from build123d import *

# Parameters (mm, degrees)
PAD_DEPTH          = 1.5
SKETCH001_R        = 2.9
PAD001_DEPTH       = 2
SKETCH002_R        = 2.35
POCKET_DEPTH       = 2.6
SKETCH003_R        = 0.75
POCKET001_DEPTH    = 0.901
SKETCH004_R        = 2.9
PAD002_DEPTH       = 1
SKETCH005_R        = 2.05
POCKET002_DEPTH    = 1
SKETCH006_R        = 0.5
POCKET003_DEPTH    = 74.221011
POLARPATTERN_COUNT = 4


with BuildPart() as part:
    # Sketch → Pad (new body)
    with BuildSketch(Plane.XY):
        with BuildLine():
            ThreePointArc((-10.573077, 1.992497), (-12.4, 0), (-10.573077, -1.992497))
            Line((-10.573077, -1.992497), (-3.096776, -2.641921))
            ThreePointArc((-2.641921, -3.096776), (-2.786492, -2.786492), (-3.096776, -2.641921))
            Line((-1.992497, -10.573077), (-2.641921, -3.096776))
            ThreePointArc((-1.992497, -10.573077), (0, -12.4), (1.992497, -10.573077))
            Line((2.641921, -3.096776), (1.992497, -10.573077))
            ThreePointArc((3.096776, -2.641921), (2.786492, -2.786492), (2.641921, -3.096776))
            Line((3.096776, -2.641921), (10.573077, -1.992497))
            ThreePointArc((10.573077, -1.992497), (12.4, 0), (10.573077, 1.992497))
            Line((10.573077, 1.992497), (3.096776, 2.641921))
            ThreePointArc((2.641921, 3.096776), (2.786492, 2.786492), (3.096776, 2.641921))
            Line((1.992497, 10.573077), (2.641921, 3.096776))
            ThreePointArc((1.992497, 10.573077), (0, 12.4), (-1.992497, 10.573077))
            Line((-1.992497, 10.573077), (-2.641921, 3.096776))
            ThreePointArc((-3.096776, 2.641921), (-2.786492, 2.786492), (-2.641921, 3.096776))
            Line((-10.573077, 1.992497), (-3.096776, 2.641921))
        make_face()
    extrude(amount=PAD_DEPTH)

    # Sketch001 → Pad001 (new body)
    with BuildSketch(Plane.XY.offset(1.5)):
        Circle(SKETCH001_R)
    extrude(amount=PAD001_DEPTH)

    # Sketch002 → Pocket (cut)
    with BuildSketch(Plane.XY.offset(3.5)):
        Circle(SKETCH002_R)
    extrude(amount=-POCKET_DEPTH, mode=Mode.SUBTRACT)

    # Sketch003 → Pocket001 (cut, through all)
    with BuildSketch(Plane.XY.offset(0.9)):
        Circle(SKETCH003_R)
    extrude(amount=-POCKET001_DEPTH, mode=Mode.SUBTRACT)

    # Sketch004 → Pad002 (new body)
    with BuildSketch(Plane(origin=(0, 0, 0), x_dir=(1, 0, 0), z_dir=(0, 0, -1))):
        Circle(SKETCH004_R)
    extrude(amount=PAD002_DEPTH)

    # Sketch005 → Pocket002 (cut)
    with BuildSketch(Plane(origin=(0, 0, -1), x_dir=(1, 0, 0), z_dir=(0, 0, -1))):
        Circle(SKETCH005_R)
    extrude(amount=-POCKET002_DEPTH, mode=Mode.SUBTRACT)

    # Sketch006 → Pocket003 (cut, through all)
    with BuildSketch(Plane(origin=(0, 0, 0), x_dir=(1, 0, 0), z_dir=(0, 0, -1))):
        with Locations((-6.45, 0)):
            Circle(SKETCH006_R)
        with Locations((-9.85, 0)):
            Circle(SKETCH006_R)
    pocket003 = extrude(amount=-POCKET003_DEPTH, mode=Mode.SUBTRACT)

    # PolarPattern: Pocket003 ×4 about axis
    polarpattern_axis = Axis((0, 0, 0), (0, 0, -1))
    for i in range(1, POLARPATTERN_COUNT):
        add(pocket003.rotate(polarpattern_axis, i * 360 / POLARPATTERN_COUNT), mode=Mode.SUBTRACT)


solid = part.part
Build history of the part. All positions in model axes, mm. A direction names the side the tool comes from. Coordinates: 2 decimals unless noted, no trailing zeros. Write each loop counter-clockwise with the first axis right and the second up, starting at its lowest first coordinate (ties: lowest second). Pieces come first, ordered by that corner, then holes.
(1) 3-axis set-ups, long thin cutter, end or side, ignore diameter. For faces 1 (the cylindrical face through (5.973, 0.15, 0.74)), 2 (the cylindrical face through (-2.9, 0.1, 2.5)), 3 (the flat face through (-3, 1, 0)): which of +Z, -Z, +X, -X, +Y, -Y reach the whole face in a straight line?
(2) Pin check, flat tips, straight feed: pin 1 Ø2 at (y, z) = (-9, 1) entering from +X; pin 2 Ø1.4 at (x, y) = (0.5, -1) entering from +Z; pin 3 Ø3 at (x, y) = (0, 0) entering from -Z. Stop position of each tip, or through.
(3) Cut at C-C on z = -0.45. List the corners of the cut face in (x, y), and give its area (3 significant figures).
(4) Cut at A-A on x = -6.45. List the corners of the cut face in (y, z).
(5) Cut at D-D on x = -1.5. List the corners of the cut face in (y, z), and give its area (3 significant figures).
(6) Mould opens along Y. For faces 4 (the cylindrical face through (-0.267, -2.033, -0.507)), 5 (the flat face through (-2.313, 6.887, 0.74)), 6 (the flat face through (-6.887, -2.313, 0.74)) say: pulls with the +Y half, pulls with the -Y half, needs draft (parallel to the pull), parting line crosses it, or undercut.
(7) Drill centre lines: line 1 (X direction, y = 0, z = -0.45); line 2 (X direction, y = -9.85, z = 1.1). Where is each one in solid material? Low to high.
Working result:
1. face 1: +Z, -Z
1. face 2: +Z
1. face 3: -Z
2. pin 1: stops at x = 2.22
2. pin 2: stops at z = 0.9
2. pin 3: stops at z = 0
3. outline: circle Ø5.8 at (0, 0); hole circle Ø4.1 at (0, 0)
3. area: 13.2 mm2
4. outline: (-2.35, 0) - (-0.5, 0) - (-0.5, 1.5) - (-2.35, 1.5) - close; (0.5, 0) - (2.35, 0) - (2.35, 1.5) - (0.5, 1.5) - close
5. outline: (-11.72, 0) - (-2.48, 0) - (-2.48, -1) - (-1.4, -1) - (-1.4, 0) - (1.4, 0) - (1.4, -1) - (2.48, -1) - (2.48, 0) - (11.72, 0) - (11.72, 1.5) - (2.48, 1.5) - (2.48, 3.5) - (1.81, 3.5) - (1.81, 0.9) - (-1.81, 0.9) - (-1.81, 3.5) - (-2.48, 3.5) - (-2.48, 1.5) - (-11.72, 1.5) - close
5. area: 37.9 mm2
6. face 4: undercut
6. face 5: pulls with the +Y half
6. face 6: pulls with the -Y half
7. line 1: x = -2.9 to -2.05, 2.05 to 2.9
7. line 2: x = -2.06 to -0.5, 0.5 to 2.06
